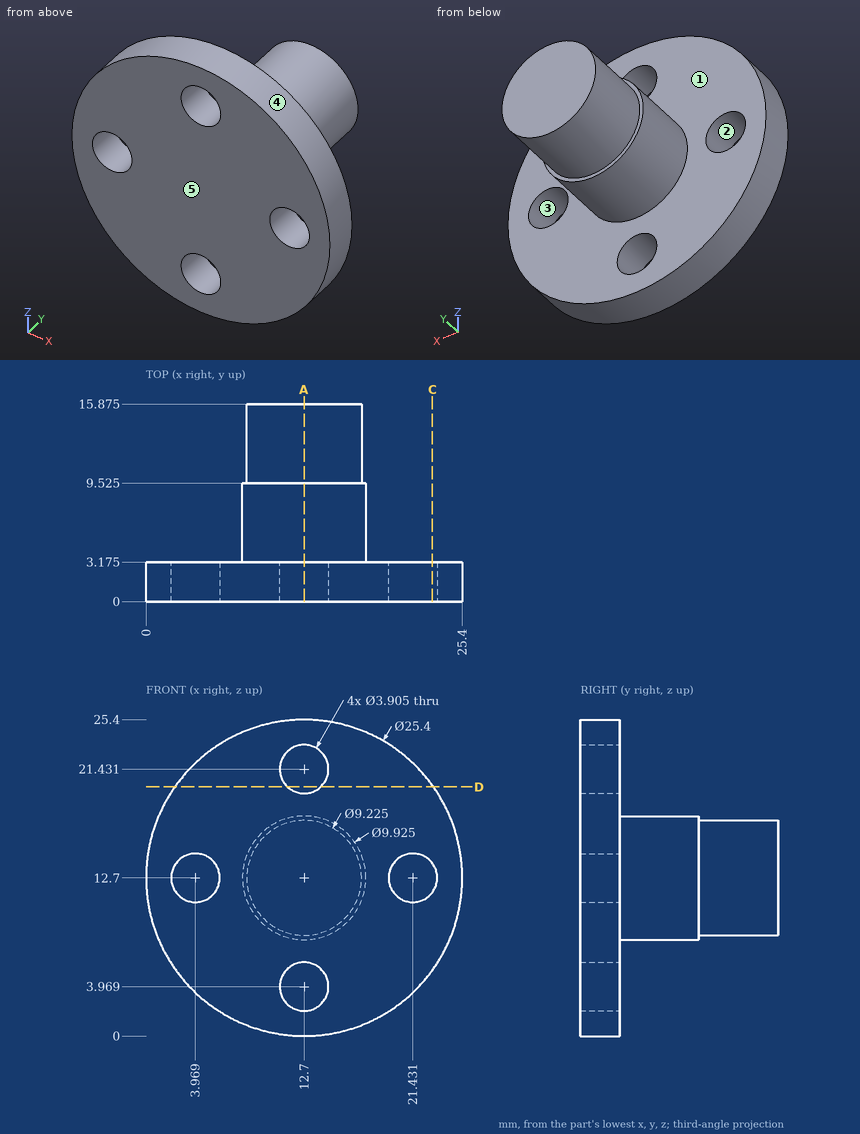
Job drawing, mm, ordinate dimensions from the low corner. One solid piece. A direction names the side the tool comes from. Round coordinates to 2 decimals unless told otherwise and drop trailing zeros. Loops run counter-clockwise (first coordinate to the right, second up) from the corner with the lowest first, then second, coordinate; pieces in that order, holes last.
Item 1: Drill centre lines: line 1 (Z direction, x = 12.7, y = 1.05); line 2 (X direction, y = 0.5, z = 12); line 3 (Y direction, x = 19, z = 16.5) (1 decimal). Where is each one in solid material? Low to high.
Item 2: Cut at A-A, the plane x = 12.7. State how many separate pieces and enclosed holes the cut face has, then the cut area to 3 significant figures.
Item 3: 3-axis set-ups, long thin cutter, end or side, ignore diameter. For the marked faces 1 and 2: which of +Z, -Z, +X, -X, +Y, -Y reach the whole face in a straight line?
Item 4: Cut at D-D, the plane z = 20. Give the cut face in (x, y) (1 decimal).
Item 5: Drop flat-ended pins along their axis: P1, Ø1.5, axis at y = 5, z = 10.5, coming from the -X side; P2, Ø6, axis at x = 12.7, z = 21.43, coming from the +Y side (3 decimals); P3, Ø5, axis at y = 2, z = 17, coming from the +X side; P4, Ø10, axis at x = 15.5, z = 15.5, coming from the -Y side. Give the stop position or say it passes through.
Item 6: Mould opens along Z. For the marked faces 3, 4 and 5 say: +Z half, -Z half, draft (parallel to the pull), parting line (faces both ways), or undercut.
Item 7: Cut at C-C, the plane x = 23. Give the cut face in (y, z) (1 decimal).
A:
1. line 1: z = 0 to 2.02, 5.92 to 19.48, 23.38 to 25.4
1. line 2: x = 0.02 to 2.15, 5.79 to 19.61, 23.25 to 25.38
1. line 3: y = 0 to 3.2
2. separate pieces: 3
2. enclosed holes: 0
2. area: 177 mm2
3. face 1: +Y
3. face 2: +Y, -Y
4. outline: (2.3, 0) - (11.4, 0) - (11.4, 3.2) - (2.3, 3.2) - close; (14, 0) - (23.1, 0) - (23.1, 3.2) - (14, 3.2) - close
5. P1: stops at x = 7.95
5. P2: stops at y = 3.175
5. P3: stops at x = 25.27
5. P4: stops at y = 0
6. face 3: undercut
6. face 4: parting line
6. face 5: draft
7. outline: (0, 5.3) - (3.2, 5.3) - (3.2, 11.5) - (0, 11.5) - close; (0, 13.9) - (3.2, 13.9) - (3.2, 20.1) - (0, 20.1) - close
